Check sheet for the modelled part. Datum: model origin and axes. Units: mm. A direction names the side the tool comes from. Coordinates: 2 decimals unless noted, no trailing zeros. Write each loop counter-clockwise with the first axis right and the second up, starting at its lowest first coordinate (ties: lowest second). Pieces come first, ordered by that corner, then holes. Notation, with made-up numbers: (62, -34) -> (87, -34) arc R22 cw to (87, -21) -> close; hole circle Ø9 at (27, 5). An arc over 180 degrees is marked (long way). One line per item, written item: value. Start each with the question number.
1) Sectioned sample at A-A on z = 27.5. Enter the section's corners in (x, y), plus the area to 3 significant figures.
2) Set-up check for faces 5 (the cylindrical face through (-18.423, 11.556, 11.778)), 6 (the flat face through (-9, 24, -5.5)), 7 (the cylindrical face through (-18.42, -11.4, 11.93)), 8 (the cylindrical face through (5, 0, -31)): record each of +Z, -Z, +X, -X, +Y, -Y from which the full face is reachable in a straight line by a thin tool's end or side.
3) Gauge pin test, flat ends, axial feed: P1, Ø20.5, axis at y = 2, z = -6, coming from the +X side; P2, Ø8, axis at x = -6, y = -27, coming from the -Z side; P3, Ø4, axis at x = -9.5, z = -3.5, coming from the +Y side; P4, Ø1.3, axis at y = 0, z = 0, coming from the +X side. Record the tip position at first contact, or that the pin passes through.
4) Scan lines: line 1 along Y through (x, z) = (-13.75, 29); line 2 along Z through (x, y) = (-16.75, 29); line 3 along X through (y, z) = (-1.5, 12.5). Record each from-to range of solid material in increasing order. Write a range as [from, to].
5) Sectioned sample at C-C on x = 3.25. Enter the section's corners in (y, z), plus the area to 3 significant figures.
6) Draft check along Z on faces 1 (the cylindrical face through (-17.67, -1.73, -7.81)), 2 (the flat face through (-9, 24, 5.5)), 3 (the flat face through (-9, 5, 24)), 4 (the cylindrical face through (-18.423, -11.556, -11.778)). Enter one of: +Z half, -Z half, draft (parallel to the pull), parting line (faces both ways), or undercut.
7) Sectioned sample at D-D on y = 21. Enter the section's corners in (x, z), plus the area to 3 significant figures.
8) Sectioned sample at B-B on y = 27.5. Enter the section's corners in (x, z), plus the area to 3 significant figures.
```python
from build123d import *
from OCP.BRepFilletAPI import BRepFilletAPI_MakeChamfer

# Parameters (mm, degrees)
BOSS_EXTRUDE1_DEPTH = 18.916428128
SKETCH3_R           = 1.15
CUT_EXTRUDE1_DEPTH  = 17.416428128
CUT_EXTRUDE3_REACH  = 51.702
SKETCH10_R          = 1.1
SKETCH8_R           = 3.5
BOSS_EXTRUDE2_DEPTH = 10
CIRPATTERN2_COUNT   = 4
CHAMFER1_SIZE       = 0.8
CHAMFER1_SIZE2      = 1.385640646


# Read off the part's stored shape, not the designer's step: Roller coating 12, Roller core 12 coated
with BuildPart() as part:
    # Roller coating 12 outline → Roller coating 12 (revolve)
    with BuildSketch(Plane.YX):
        with BuildLine():
            ThreePointArc((12.7, -17.916428128), (15.217989764, 0), (12.7, 17.916428128))
            Line((12.7, 17.916428128), (8, 17.916428128))
            Line((8, 17.916428128), (8, 17.416428128))
            Line((8, 17.416428128), (12.322080058, 17.416428128))
            ThreePointArc((12.322080058, 17.416428128), (14.717989764, 0), (12.322080058, -17.416428128))
            Line((12.322080058, -17.416428128), (8, -17.416428128))
            Line((8, -17.416428128), (8, -17.916428128))
            Line((8, -17.916428128), (12.7, -17.916428128))
        make_face()
    revolve(axis=Axis((0, 0, 0), (1, 0, 0)))


with BuildPart() as body_2:
    # Roller core 12 coated outline → Roller core 12 coated (revolve)
    with BuildSketch(Plane.YX):
        with BuildLine():
            Line((1.15, 17.416428128), (1.15, -17.416428128))
            Line((1.15, -17.416428128), (12.322080058, -17.416428128))
            ThreePointArc((12.322080058, -17.416428128), (14.717989764, 0), (12.322080058, 17.416428128))
            Line((12.322080058, 17.416428128), (1.15, 17.416428128))
        make_face()
    revolve(axis=Axis((0, 0, 0), (1, 0, 0)))


with BuildPart() as part_1:
    add(part.part)

    # Combine1: union body 2
    add(body_2.part)


with BuildPart() as body_2_2:
    # Sketch1 → Revolve1 (revolve)
    with BuildSketch(Plane.XY, mode=Mode.PRIVATE) as revolve1_sk:
        with BuildLine():
            Line((0, 0), (0, 15.217989764))
            Line((0, 15.217989764), (0, 19.017989764))
            ThreePointArc((0, 19.017989764), (-9.046251562, 18.385414232), (-17.916428128, 16.5))
            Line((-17.916428128, 16.5), (-18.916428128, 16.5))
            Line((-18.916428128, 16.5), (-18.916428128, 0))
            Line((-18.916428128, 0), (0, 0))
        make_face()
    revolve(revolve1_sk.sketch.rotate(Axis((-18.916428128, 0, 0), (1, 0, 0)), 270), axis=Axis((-18.916428128, 0, 0), (1, 0, 0)))

    # Sketch5 → Boss-Extrude1 (add)
    with BuildSketch(Plane(origin=(0, 0, 0), x_dir=(0, 0, -1), z_dir=(1, 0, 0))):
        with BuildLine():
            Line((5.5, -32.031234756), (5.5, -15.556349186))
            ThreePointArc((5.5, -15.556349186), (0, -16.5), (-5.5, -15.556349186))
            Line((-5.5, -15.556349186), (-5.5, -32.031234756))
            ThreePointArc((-5.5, -32.031234756), (0, -32.5), (5.5, -32.031234756))
        make_face()
        with BuildLine():
            Line((-5.5, 32.031234756), (-5.5, 15.556349186))
            ThreePointArc((-5.5, 15.556349186), (0, 16.5), (5.5, 15.556349186))
            Line((5.5, 15.556349186), (5.5, 32.031234756))
            ThreePointArc((5.5, 32.031234756), (0, 32.5), (-5.5, 32.031234756))
        make_face()
        with BuildLine():
            Line((32.113081447, 5), (15.724185194, 5))
            ThreePointArc((15.724185194, 5), (16.5, 0), (15.724185194, -5))
            Line((15.724185194, -5), (32.113081447, -5))
            ThreePointArc((32.113081447, -5), (32.5, 0), (32.113081447, 5))
        make_face()
        with BuildLine():
            Line((-32.113081447, -5), (-15.724185194, -5))
            ThreePointArc((-15.724185194, -5), (-16.5, 0), (-15.724185194, 5))
            Line((-15.724185194, 5), (-32.113081447, 5))
            ThreePointArc((-32.113081447, 5), (-32.5, 0), (-32.113081447, -5))
        make_face()
    extrude(amount=-BOSS_EXTRUDE1_DEPTH)

    # Combine2: cut part
    add(part_1.part, mode=Mode.SUBTRACT)

    # Sketch3 → Cut-Extrude1 (cut)
    with BuildSketch(Plane(origin=(0, 0, 0), x_dir=(0, 0, -1), z_dir=(1, 0, 0))):
        Circle(SKETCH3_R)
    extrude(amount=-CUT_EXTRUDE1_DEPTH, mode=Mode.SUBTRACT)

    # Sketch10 → Cut-Extrude3 (cut, up to next)
    with BuildSketch(Plane(origin=(0, 0, 0), x_dir=(0, 0, -1), z_dir=(1, 0, 0)), mode=Mode.PRIVATE) as cut_extrude3_sk1:
        Circle(SKETCH10_R)
    cut_extrude3_tool1 = extrude(cut_extrude3_sk1.sketch, amount=-CUT_EXTRUDE3_REACH, mode=Mode.PRIVATE) & body_2_2.part
    add(cut_extrude3_tool1.solids().sort_by_distance((0, 0, 0))[0], mode=Mode.SUBTRACT)

    # Sketch4 → Revolve2 (revolve)
    with BuildSketch(Plane.XY, mode=Mode.PRIVATE) as revolve2_sk:
        Polygon((0, 18.216989764), (0.8, 17.117989764), (0, 16.018989764), align=None)
    revolve(revolve2_sk.sketch.rotate(Axis((-18.916428128, 0, 0), (1, 0, 0)), 90), axis=Axis((-18.916428128, 0, 0), (1, 0, 0)))

    # Sketch8 → Boss-Extrude2 (add)
    with BuildSketch(Plane(origin=(0, 0, 0), x_dir=(0, 0, -1), z_dir=(1, 0, 0))):
        with Locations(Location((0, -27.5, 0), (0, 0, 180))):
            Circle(SKETCH8_R)
    boss_extrude2 = extrude(amount=BOSS_EXTRUDE2_DEPTH)

    # CirPattern2: Boss-Extrude2 ×4 about axis
    cirpattern2_axis = Axis((0, 0, 0), (1, 0, 0))
    for i in range(1, CIRPATTERN2_COUNT):
        add(boss_extrude2.rotate(cirpattern2_axis, i * 360 / CIRPATTERN2_COUNT))

    # Chamfer1: one chamfer whose edges measure the first distance from different faces: ONE call of the kernel's chamfer builder (chamfer() names one face for all edges)
    chamfer1_edges_1 = [body_2_2.edges().sort_by_distance(p)[0] for p in [
        (0, -32.5, 0),
    ]]
    chamfer1_side_1 = [body_2_2.faces().sort_by_distance(p)[0] for p in [
        (-9.458214064, -32.5, 0),
    ]]
    chamfer1_edges_2 = [body_2_2.edges().sort_by_distance(p)[0] for p in [
        (0, 0, -32.5),
    ]]
    chamfer1_side_2 = [body_2_2.faces().sort_by_distance(p)[0] for p in [
        (-9.458214064, 0, -32.5),
    ]]
    chamfer1_edges_3 = [body_2_2.edges().sort_by_distance(p)[0] for p in [
        (0, 32.5, 0),
    ]]
    chamfer1_side_3 = [body_2_2.faces().sort_by_distance(p)[0] for p in [
        (-9.458214064, 32.5, 0),
    ]]
    chamfer1_edges_4 = [body_2_2.edges().sort_by_distance(p)[0] for p in [
        (0, 0, 32.5),
    ]]
    chamfer1_side_4 = [body_2_2.faces().sort_by_distance(p)[0] for p in [
        (-9.458214064, 0, 32.5),
    ]]
    chamfer1 = BRepFilletAPI_MakeChamfer(body_2_2.part.solid().wrapped)
    for e in chamfer1_edges_1:
        chamfer1.Add(CHAMFER1_SIZE, CHAMFER1_SIZE2, e.wrapped, chamfer1_side_1[0].wrapped)  # the first distance lies on this face
    for e in chamfer1_edges_2:
        chamfer1.Add(CHAMFER1_SIZE, CHAMFER1_SIZE2, e.wrapped, chamfer1_side_2[0].wrapped)  # the first distance lies on this face
    for e in chamfer1_edges_3:
        chamfer1.Add(CHAMFER1_SIZE, CHAMFER1_SIZE2, e.wrapped, chamfer1_side_3[0].wrapped)  # the first distance lies on this face
    for e in chamfer1_edges_4:
        chamfer1.Add(CHAMFER1_SIZE, CHAMFER1_SIZE2, e.wrapped, chamfer1_side_4[0].wrapped)  # the first distance lies on this face
    add(Compound.cast(chamfer1.Shape()), mode=Mode.REPLACE)


solid = body_2_2.part
```
Answers:
1. outline: (-18.92, -5) -> (0, -5) -> (0, -3.5) -> (10, -3.5) -> (10, 3.5) -> (0, 3.5) -> (0, 5) -> (-18.92, 5) -> close
1. area: 259 mm2
2. face 5: +Z, -X, +Y
2. face 6: -Z, -X, +Y
2. face 7: +Z, -X, -Y
2. face 8: +X
3. P1: stops at x = 0.4
3. P2: stops at z = -5.5
3. P3: stops at y = 32.47
3. P4: passes through
4. line 1: y = [-5, 5]
4. line 2: z = [-5.5, 5.5]
4. line 3: x = [-18.92, -17.92]
5. outline: circle Ø7 at (-27.5, 0); circle Ø7 at (0, -27.5); circle Ø7 at (0, 27.5); circle Ø7 at (27.5, 0)
5. area: 154 mm2
6. face 1: undercut
6. face 2: +Z half
6. face 3: draft
6. face 4: -Z half
7. outline: (-18.92, -5.5) -> (0, -5.5) -> (0, 5.5) -> (-18.92, 5.5) -> close
7. area: 208 mm2
8. outline: (-18.92, -5.5) -> (0, -5.5) -> (0, -3.5) -> (10, -3.5) -> (10, 3.5) -> (0, 3.5) -> (0, 5.5) -> (-18.92, 5.5) -> close
8. area: 278 mm2
